```python
from build123d import *

# Parameters (mm, degrees)
SKETCH10_W               = 35
SKETCH10_H               = 20
BOSS_EXTRUDE9_DEPTH      = 6.5
SKETCH11_W               = 7
SKETCH11_H               = 15
CUT_EXTRUDE4_DEPTH       = 1
CUT_EXTRUDE4_DEPTH_BACK  = 36
BOSS_EXTRUDE10_DEPTH     = 2.5
CUT_EXTRUDE5_DEPTH       = 20
CUT_EXTRUDE6_DEPTH       = 20
BOSS_EXTRUDE11_DEPTH     = 10
SKETCH23_R               = 1.5
CUT_EXTRUDE7_DEPTH       = 34
SKETCH25_R               = 1.5
BOSS_EXTRUDE12_DEPTH     = 12.5
SKETCH27_W               = 7
SKETCH27_H               = 15
CUT_EXTRUDE9_DEPTH       = 20
SKETCH28_W               = 7
SKETCH28_H               = 6.245605743
CUT_EXTRUDE10_DEPTH      = 20
BOSS_EXTRUDE13_DEPTH     = 2.5
BOSS_EXTRUDE14_DEPTH     = 5
SKETCH31_R               = 2.5
CUT_EXTRUDE11_DEPTH      = 44.363432005
CUT_EXTRUDE11_DEPTH_BACK = 111.559122284


with BuildPart() as part:
    # Sketch10 → Boss-Extrude9 (new body, symmetric)
    with BuildSketch(Plane.XY):
        Rectangle(SKETCH10_W, SKETCH10_H)
    extrude(amount=BOSS_EXTRUDE9_DEPTH, both=True)

    # Sketch11 → Cut-Extrude4 (cut, two sides)
    with BuildSketch(Plane.ZY.offset(17.5)) as cut_extrude4_sk:
        with Locations((0, 2.5)):
            Rectangle(SKETCH11_W, SKETCH11_H)
    extrude(amount=CUT_EXTRUDE4_DEPTH, mode=Mode.SUBTRACT)
    extrude(cut_extrude4_sk.sketch, amount=-CUT_EXTRUDE4_DEPTH_BACK, mode=Mode.SUBTRACT)

    # Sketch19 → Boss-Extrude10 (add, symmetric)
    with BuildSketch(Plane(origin=(7.588283472, -8.408592155, 0), x_dir=(-0.742391283, -0.669966553, 0), z_dir=(0.669966553, -0.742391283, 0))):
        Polygon((-6.806611372, 12.5), (-6.806611372, 6.5), (5.959262629, 6.5), (5.959262629, -6.5), (-9.021371158, -6.5), (-9.021371158, -14.5), (143.193388628, 27.210594591), (143.193388628, 47.516269419), align=None)
        Polygon((23.416933748, 15.447357766), (23.416933748, -2.932626146), (48.137832442, 21.788272547), align=None, mode=Mode.SUBTRACT)
        Polygon((34.103204957, 0), (57.455439154, 23.352234198), (87.138773177, 15.447357766), align=None, mode=Mode.SUBTRACT)
        Polygon((69.571415231, 26.355349278), (96.907086696, 19.075671565), (112.271299908, 37.384757918), align=None, mode=Mode.SUBTRACT)
        Polygon((116.606735087, 37.384757918), (103.00206527, 19.075671565), (136.676990559, 28.230214742), (136.676990559, 43.712984767), align=None, mode=Mode.SUBTRACT)
    boss_extrude10 = extrude(amount=BOSS_EXTRUDE10_DEPTH, both=True)

    # Mirror3: Boss-Extrude10 across plane
    add(boss_extrude10.mirror(Plane(origin=(0, 0, 0), x_dir=(0, 0, 1), z_dir=(-0.707106781, 0.707106781, 0))))

    # Sketch20 → Cut-Extrude5 (cut)
    with BuildSketch(Plane(origin=(0, 0, -6.5), x_dir=(-1, 0, 0), z_dir=(0, 0, -1))):
        Polygon((-13.528185403, -10), (16.011199993, 15.429392684), (-17.5, 15.429392684), (-17.5, -10), align=None)
    extrude(amount=CUT_EXTRUDE5_DEPTH, mode=Mode.SUBTRACT)

    # Sketch21 → Cut-Extrude6 (cut)
    with BuildSketch(Plane.XY.offset(6.5)):
        Polygon((-16.011199993, 15.429392684), (13.528185403, -10), (17.5, -10), (17.5, 17.942203717), align=None)
    extrude(amount=CUT_EXTRUDE6_DEPTH, mode=Mode.SUBTRACT)

    # Sketch22 → Boss-Extrude11 (add)
    with BuildSketch(Plane(origin=(0, 0, -6.5), x_dir=(-1, 0, 0), z_dir=(0, 0, -1))):
        Polygon((-4.751258092, -14.336345099), (15.731654079, 3.20511341), (9.645399477, 9.949304357), (-11.495449039, -8.250090497), align=None)
    boss_extrude11 = extrude(amount=BOSS_EXTRUDE11_DEPTH)

    # Mirror5: Boss-Extrude11 across plane
    add(boss_extrude11.mirror(Plane.XY))

    # Sketch23 → Cut-Extrude7 (cut, through all)
    with BuildSketch(Plane(origin=(0, 0, -16.5), x_dir=(-1, 0, 0), z_dir=(0, 0, -1))):
        with Locations((2.661358897, -1.787066196)):
            Circle(SKETCH23_R)
    extrude(amount=-CUT_EXTRUDE7_DEPTH, mode=Mode.SUBTRACT)

    # Sketch25 → Boss-Extrude12 (add, symmetric)
    with BuildSketch(Plane.XY.offset(-37.363432005)):
        Polygon((-110.446046435, -140.151182494), (-82.161775188, -111.866911247), (-110.446046435, -83.582639999), (-138.730317683, -111.866911247), align=None)
        with Locations((-110.446046435, -93.482134936)):
            Circle(SKETCH25_R, mode=Mode.SUBTRACT)
        with Locations((-92.061270124, -111.866911247)):
            Circle(SKETCH25_R, mode=Mode.SUBTRACT)
        with Locations((-110.446046435, -130.251687558)):
            Circle(SKETCH25_R, mode=Mode.SUBTRACT)
        with Locations((-128.830822746, -111.866911247)):
            Circle(SKETCH25_R, mode=Mode.SUBTRACT)
    extrude(amount=BOSS_EXTRUDE12_DEPTH, both=True)

    # Sketch27 → Cut-Extrude9 (cut)
    with BuildSketch(Plane.ZY.offset(17.5)):
        with Locations((0, 2.5)):
            Rectangle(SKETCH27_W, SKETCH27_H)
    extrude(amount=-CUT_EXTRUDE9_DEPTH, mode=Mode.SUBTRACT)

    # Sketch28 → Cut-Extrude10 (cut)
    with BuildSketch(Plane(origin=(-17.5, 0, 0), x_dir=(0, 0, -1), z_dir=(1, 0, 0))):
        with Locations((0, -1.877197128)):
            Rectangle(SKETCH28_W, SKETCH28_H)
    extrude(amount=-CUT_EXTRUDE10_DEPTH, mode=Mode.SUBTRACT)

    # Sketch29 → Boss-Extrude13 (add, symmetric)
    with BuildSketch(Plane(origin=(0.710432406, -0.710432406, 0), x_dir=(0, 0, -1), z_dir=(0.707106781, -0.707106781, 0))):
        Polygon((-19.348604545, -180.98841896), (25.940877716, -162.519522981), (25.940877716, -150.294032198), (-9.701797277, -150.294032198), (-104.059122284, -136.781099823), (-104.059122284, -145.835191948), align=None)
        Polygon((-86.194464325, -143.014000871), (-85.469075751, -150.294032198), (-60.635525341, -147.819595909), align=None, mode=Mode.SUBTRACT)
        Polygon((-77.244001552, -152.888925889), (-36.176017731, -169.28301403), (-51.201535414, -150.294032198), align=None, mode=Mode.SUBTRACT)
        Polygon((15.288083197, -155.48381958), (-9.701797277, -155.48381958), (-16.926790753, -176.046505079), (15.288083197, -162.519522981), align=None, mode=Mode.SUBTRACT)
        Polygon((-23.96640174, -175.703793654), (-44.343704752, -149.951320773), (-16.741408265, -155.141108155), align=None, mode=Mode.SUBTRACT)
        Polygon((25.940877716, -162.519522981), (25.940877716, -150.294032198), (-9.701797277, -150.294032198), (-104.059122284, -136.781099823), (-104.059122284, -145.835191948), (-19.348604545, -180.98841896), align=None)
        Polygon((-51.201535414, -150.294032198), (-36.176017731, -169.28301403), (-77.244001552, -152.888925889), align=None, mode=Mode.SUBTRACT)
        Polygon((-44.343704752, -149.951320773), (-16.741408265, -155.141108155), (-23.96640174, -175.703793654), align=None, mode=Mode.SUBTRACT)
        Polygon((-16.926790753, -176.046505079), (-9.701797277, -155.48381958), (15.288083197, -155.48381958), (15.288083197, -162.519522981), align=None, mode=Mode.SUBTRACT)
        Polygon((-60.635525341, -147.819595909), (-85.469075751, -150.294032198), (-86.194464325, -143.014000871), align=None, mode=Mode.SUBTRACT)
    extrude(amount=BOSS_EXTRUDE13_DEPTH, both=True)

    # Sketch30 → Boss-Extrude14 (add)
    with BuildSketch(Plane(origin=(2.478199359, -2.478199359, 0), x_dir=(0, 0, -1), z_dir=(0.707106781, -0.707106781, 0))):
        Polygon((-41.059122284, -146.781099823), (-2.200668351, -12.59179888), (-4.968563169, -11.790273627), (-44.059122284, -146.781099823), align=None)
    extrude(amount=-BOSS_EXTRUDE14_DEPTH)

    # Sketch31 → Cut-Extrude11 (cut, two sides)
    with BuildSketch(Plane(origin=(0, 0, -6.5), x_dir=(-1, 0, 0), z_dir=(0, 0, -1))) as cut_extrude11_sk:
        with Locations((-12.5, 5)):
            Circle(SKETCH31_R)
    extrude(amount=CUT_EXTRUDE11_DEPTH, mode=Mode.SUBTRACT)
    extrude(cut_extrude11_sk.sketch, amount=-CUT_EXTRUDE11_DEPTH_BACK, mode=Mode.SUBTRACT)


solid = part.part
```
The model under review builds one solid part; all positions refer to its coordinate system, in mm. A direction names the side the tool comes from. Round coordinates to 2 decimals unless told otherwise and drop trailing zeros. Loops run counter-clockwise (first coordinate to the right, second up) from the corner with the lowest first, then second, coordinate; pieces in that order, holes last.
1) Consider section A-A on z = 46.5. State the section outline as (x, y) points.
Values follow:
outline: (-121.07, -118.95) - (-117.53, -122.49) - (-114.31, -119.27) - (-117.84, -115.73) - close; (-111.53, -109.42) - (-108, -112.95) - (-100.07, -105.03) - (-103.6, -101.49) - close
2) Tool access review of faces 4 (the face through (-1, -1, -16.5)), 5 (the face through (-102.1, -103.5, 73.6)), 6 (the face through (-99.084, -100.555, 73.441)): name each direction out of +Z, -Z, +X, -X, +Y, -Y from which nothing blocks a thin tool from reaching the whole face with its end or side.
Values follow:
face 4: -Z, +X, +Y
face 5: none
face 6: +X, +Y
3) Clearance check with flat-ended pins moving along their axes: P1, Ø5, axis at x = -8, y = -3.5, coming from the +Z side; P2, Ø1.1, axis at y = -8, z = 3, coming from the -X side; P3, Ø9.5, axis at x = -110, y = -112, coming from the +Z side. State where each tip first meets the part, or that it passes through.
Values follow:
P1: stops at z = 16.5
P2: stops at x = -26.34
P3: stops at z = 88.65
4) Wall thickness on line 1 along Y through (x, z) = (12, 5); line 2 along Z through (x, y) = (-93, -115.5); line 3 along X through (y, z) = (-106, -2.5): over which ranges is each line inside the solid? List them lowest first.
Values follow:
line 1: y = -10 to 2.55, 7.45 to 10
line 2: z = -49.86 to -24.86
line 3: x = -108.11 to -106.55
5) The part is to be moulded in two halves that separate along Z. For faces 1 (the face through (-46.151, -56.952, -30.994)), 2 (the face through (4, 2, 6.5)), 3 (the face through (-69.955, -78.434, -28.102)), say which applies: pulls with the +Z half, pulls with the -Z half, needs draft (parallel to the pull), parting line crosses it, or undercut.
Values follow:
face 1: pulls with the -Z half
face 2: pulls with the +Z half
face 3: undercut
